Could you check a few things on this model? Use its own coordinates, in mm. A direction names the side the tool comes from. Coordinates: 2 decimals unless noted, no trailing zeros. Order: outer loops, then holes, each group sorted by start corner. A loop starts at its lowest first (then second) coordinate and runs counter-clockwise, first axis right, second up. Notation, with made-up numbers: (39.25, 70) -> (97.25, 70) arc R16 ccw to (97.25, 99) -> close; hole circle Ø2 at (7.5, 57.5). An arc over 180 degrees is marked (long way). Return JSON: item names as keys, results as strings. Group by question number.
from build123d import *

# Parameters (mm, degrees)
CYLINDER001_R            = 2
CYLINDER001_DEPTH        = 10
CYLINDER_W               = 25
CYLINDER_H               = 5
CYLINDER_ANGLE           = 270
CYLINDER_PLACEMENT_ANGLE = 45


with BuildPart() as cilindre001:
    # Cylinder001 → Cylinder001 (new body)
    with BuildSketch(Plane(origin=(0, 10, -2), x_dir=(1, 0, 0), z_dir=(0, 0, 1))):
        Circle(CYLINDER001_R)
    extrude(amount=CYLINDER001_DEPTH)


with BuildPart() as cut:
    # Cylinder → Cylinder (revolve)
    with BuildSketch(Plane.XZ):
        with Locations((12.5, 2.5)):
            Rectangle(CYLINDER_W, CYLINDER_H)
    revolve(axis=Axis((0, 0, 0), (0, 0, 1)), revolution_arc=CYLINDER_ANGLE)


with BuildPart() as cut_1:
    # Cylinder placement: moved
    add(cut.part.rotate(Axis((0, 0, 0), (0, 0, 1)), CYLINDER_PLACEMENT_ANGLE))

    # Cut: cut Cilindre001
    add(cilindre001.part, mode=Mode.SUBTRACT)


solid = cut_1.part
Q1. I need wall thicknesses on line 1 along Y through (x, z) = (10, 3.8); line 2 along X through (y, z) = (10, 2.1); line 3 along Y through (x, z) = (13, 1.2). Which ranges of each line are inside material? Lowest first, please. Write a range as from..to.
Q2. I want a section at D-D on y = -5. Please give me the cut outline in (x, z), and give its area (3 significant figures).
Q3. We'd pull the mould along X, two halves only. Please class faces 3 (the cylindrical face through (-24.986, 0.825, 2.535)), 4 (the flat face through (-8, 0, 5)), 5 (the flat face through (9, -9, 3)), 6 (the cylindrical face through (0, 12, 2)): pulls with the +X half, pulls with the -X half, needs draft (parallel to the pull), parting line crosses it, or undercut.
Q4. I want a section at B-B on y = 10. Please give me the cut outline in (x, z).
Q5. I'm going to push a flat-ended pin straight in: pin 1 Ø2 at (y, z) = (7.5, 4) entering from -X. Where does the tip first touch, or does it pass through?
Q6. I want a section at A-A on x = 4. Please give me the cut outline in (y, z).
Q7. I want a section at C-C on z = 0.7. Please give me the cut outline in (x, y).
Q8. On a 3-axis mill with a long thin cutter (end or side, diameter ignored), from which of +Z, -Z, +X, -X, +Y, -Y can I reach the whole of each face in a straight line? I mean faces 1 (the flat face through (9, 9, 3)), 2 (the flat face through (-8, 0, 0)). Say none if no direction works.
Response values:
{
 "1": {"line 1": "y = -22.91..-10, 10..22.91", "line 2": "x = -22.91..-2, 2..10", "line 3": "y = -21.35..-13, 13..21.35"},
 "2": {"outline": "(-24.49, 0) -> (5, 0) -> (5, 5) -> (-24.49, 5) -> close", "area": "147 mm²"},
 "3": {"face 3": "parting line crosses it", "face 4": "needs draft", "face 5": "pulls with the +X half", "face 6": "undercut"},
 "4": {"outline": "(-22.91, 0) -> (-2, 0) -> (-2, 5) -> (-22.91, 5) -> close; (2, 0) -> (10, 0) -> (10, 5) -> (2, 5) -> close"},
 "5": {"pin 1": "stops at x = -24.14"},
 "6": {"outline": "(-24.68, 0) -> (-4, 0) -> (-4, 5) -> (-24.68, 5) -> close; (4, 0) -> (24.68, 0) -> (24.68, 5) -> (4, 5) -> close"},
 "7": {"outline": "(0, 0) -> (17.68, 17.68) arc R25 ccw (long way) to (17.68, -17.68) -> close; hole circle Ø4 at (0, 10)"},
 "8": {"face 1": "+Z, -Z, +X", "face 2": "-Z, +X, -X, +Y, -Y"}
}
